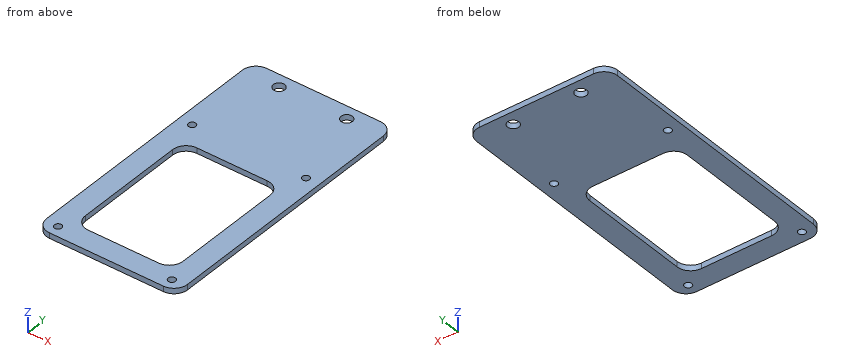
```python
from build123d import *

# Parameters (mm, degrees)
SKETCH_1_W          = 52
SKETCH_1_H          = 102
EXTRUDE_1_DEPTH     = 2
FILLET_1_R          = 5
SKETCH_2_R          = 2.1
SKETCH_2_R_2        = 1.35
CUT_EXTRUDE_1_DEPTH = 3
SKETCH_3_W          = 36
SKETCH_3_H          = 51
CUT_EXTRUDE_2_DEPTH = 10
FILLET_2_R          = 5


with BuildPart() as part:
    # 草图1 → 凸台-拉伸1 (new body)
    with BuildSketch(Plane.XY):
        Rectangle(SKETCH_1_W, SKETCH_1_H)
    extrude(amount=EXTRUDE_1_DEPTH)

    # 圆角1
    fillet_1_edges = [part.edges().sort_by_distance(p)[0] for p in [
        (26, -51, 1),
        (-26, -51, 1),
        (-26, 51, 1),
        (26, 51, 1),
    ]]
    fillet(fillet_1_edges, radius=FILLET_1_R)

    # 草图2 → 切除-拉伸1 (cut, through all)
    with BuildSketch(Plane.XY.offset(2)):
        with Locations((-12.5, 46)):
            Circle(SKETCH_2_R)
        with Locations((12.5, 46)):
            Circle(SKETCH_2_R)
        with Locations((-21, 16)):
            Circle(SKETCH_2_R_2)
        with Locations((21, 16)):
            Circle(SKETCH_2_R_2)
        with Locations((-21, -47)):
            Circle(SKETCH_2_R_2)
        with Locations((21, -47)):
            Circle(SKETCH_2_R_2)
    extrude(amount=-CUT_EXTRUDE_1_DEPTH, mode=Mode.SUBTRACT)

    # 草图3 → 切除-拉伸2 (cut)
    with BuildSketch(Plane.XY.offset(2)):
        with Locations((0, -17.5)):
            Rectangle(SKETCH_3_W, SKETCH_3_H)
    extrude(amount=-CUT_EXTRUDE_2_DEPTH, mode=Mode.SUBTRACT)

    # 圆角2
    fillet_2_edges = [part.edges().sort_by_distance(p)[0] for p in [
        (18, 8, 1),
        (18, -43, 1),
        (-18, -43, 1),
        (-18, 8, 1),
    ]]
    fillet(fillet_2_edges, radius=FILLET_2_R)


solid = part.part
```
Verification items for the finished model (mm, model axes). Coordinates: 2 decimals unless noted, no trailing zeros. Loops run counter-clockwise (first coordinate to the right, second up) from the corner with the lowest first, then second, coordinate; pieces in that order, holes last. Notation, with made-up numbers: (2.25, -32) -> (19.25, -32) arc R17 ccw to (19.25, -22) -> close; hole circle Ø7 at (-4, 12). An arc over 180 degrees is marked (long way). Answer in a Markdown table with one row per item. Add a question column.
1. Section check D-D, the plane y = 16. Enter the section's corners in (x, z).
2. Section check B-B, the plane x = 8.5. Enter the section's corners in (y, z), then the cut area to 3 significant figures.
3. Section check A-A, the plane y = -6.5. Enter the section's corners in (x, z).
4. Section check C-C, the plane z = 1.55. Enter the section's corners in (x, y).
5. Material ranges on probe 1 along Y at (x, z) = (21, 1.3); probe 2 along Y at (x, z) = (-12.5, 0.9); probe 3 along Y at (x, z) = (-1, 1.2), recorded low to high. Write a range as [from, to].
Derived:
| question | item | result |
|---|---|---|
| 1 | outline | (-26, 0) -> (-22.35, 0) -> (-22.35, 2) -> (-26, 2) -> close; (-19.65, 0) -> (19.65, 0) -> (19.65, 2) -> (-19.65, 2) -> close; (22.35, 0) -> (26, 0) -> (26, 2) -> (22.35, 2) -> close |
| 2 | outline | (-51, 0) -> (-43, 0) -> (-43, 2) -> (-51, 2) -> close; (8, 0) -> (51, 0) -> (51, 2) -> (8, 2) -> close |
| 2 | area | 102 mm² |
| 3 | outline | (-26, 0) -> (-18, 0) -> (-18, 2) -> (-26, 2) -> close; (18, 0) -> (26, 0) -> (26, 2) -> (18, 2) -> close |
| 4 | outline | (-26, -46) arc R5 ccw to (-21, -51) -> (21, -51) arc R5 ccw to (26, -46) -> (26, 46) arc R5 ccw to (21, 51) -> (-21, 51) arc R5 ccw to (-26, 46) -> close; hole circle Ø2.7 at (-21, -47); hole circle Ø2.7 at (-21, 16); hole (-18, -38) arc R5 ccw to (-13, -43) -> (13, -43) arc R5 ccw to (18, -38) -> (18, 3) arc R5 ccw to (13, 8) -> (-13, 8) arc R5 ccw to (-18, 3) -> close; hole circle Ø4.2 at (-12.5, 46); hole circle Ø4.2 at (12.5, 46); hole circle Ø2.7 at (21, -47); hole circle Ø2.7 at (21, 16) |
| 5 | probe 1 | y = [-51, -48.35], [-45.65, 14.65], [17.35, 51] |
| 5 | probe 2 | y = [-51, -43], [8, 43.9], [48.1, 51] |
| 5 | probe 3 | y = [-51, -43], [8, 51] |
